The model under review builds one solid part; all positions refer to its coordinate system, in mm. Face numbers are marked on the shaded views. Give positions to 0.01 mm unless a question says otherwise; leave off trailing zeros. Loops run counter-clockwise (first coordinate to the right, second up) from the corner with the lowest first, then second, coordinate; pieces in that order, holes last. Notation, with made-up numbers: M -34.5,61 L -15.5,61 A16 ccw -15.5,91 Z; hole C -6.75,80.5 d9. An arc over 180 degrees is marked long. Return JSON: item names as keys, results as strings.
```python
from build123d import *

# Parameters (mm, degrees)
F1_DEPTH = 203.2
F2_R     = 3.3782
F3_DEPTH = 3.175
F4_R     = 2.5527
F5_DEPTH = 3.175
F6_R     = 1.259666


with BuildPart() as f1:
    # F0 (on Front) → F1 (new body)
    with BuildSketch(Plane.XZ):
        Polygon((30.434872, 0), (0, 0), (21.520704, 21.520704), (19.27564, 23.765768), (-7.665128, -3.175), (30.434872, -3.175), align=None)
    extrude(amount=F1_DEPTH)

    # F2 (on face) → F3 (cut, through all)
    with BuildSketch(Plane(origin=(-2.245064, 0, 2.245064), x_dir=(0, -1, 0), z_dir=(-0.707107, 0, 0.707107))):
        with Locations((50.8, 11.384872)):
            Circle(F2_R)
        with Locations((152.4, 11.384872)):
            Circle(F2_R)
    extrude(amount=-F3_DEPTH, mode=Mode.SUBTRACT)

    # F4 (on face) → F5 (cut, through all)
    with BuildSketch(Plane(origin=(0, 0, -3.175), x_dir=(1, 0, 0), z_dir=(0, 0, -1))):
        with Locations((17.734872, 152.4)):
            Circle(F4_R)
        with Locations((17.734872, 50.8)):
            Circle(F4_R)
    extrude(amount=-F5_DEPTH, mode=Mode.SUBTRACT)

    # F6
    f6_edges = [f1.edges().sort_by_distance(p)[0] for p in [
        (-7.665128, -101.6, -3.175),
    ]]
    fillet(f6_edges, radius=F6_R)


solid = f1.part
```
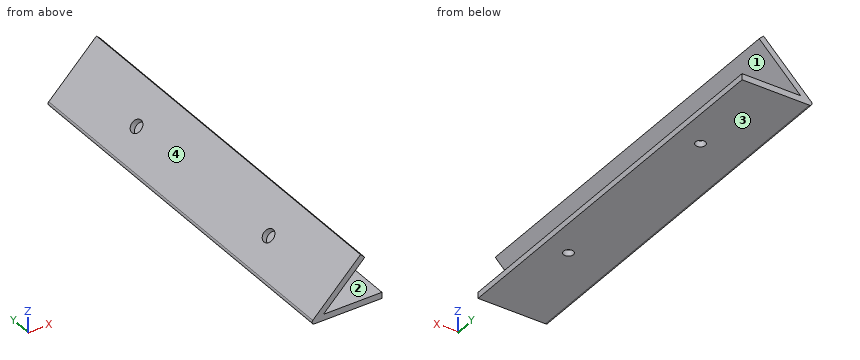
1) Consider section A-A on x = 13.5. Write out the cut boundary in (y, z) (3 decimals).
From the geometry:
{"outline": "M -203.2,-3.175 L 0,-3.175 L 0,0 L -203.2,0 Z; M -203.2,13.5 L 0,13.5 L 0,17.99 L -203.2,17.99 Z"}
2) Consider section C-C on y = -152.4. Write out the cut boundary in (x, z) (1 decimal).
From the geometry:
{"outline": "M -5.5,-1 A1.3 ccw -4.6,-3.2 L 15.2,-3.2 L 15.2,0 L 0,0 L 5.7,5.7 L 3.4,7.9 Z; M 8.2,12.7 L 10.4,10.4 L 21.5,21.5 L 19.3,23.8 Z; M 20.3,-3.2 L 30.4,-3.2 L 30.4,0 L 20.3,0 Z"}
3) Insertion check: pin 1 (1 mm diameter, centred on x = 3, z = 10.5, fed in from +Y); pin 2 (6 mm diameter, centred on y = -137, z = 5.5, fed in from +X); pin 3 (3 mm diameter, centred on y = -58, z = 6.5, fed in from -X); pin 4 (6 mm diameter, centred on y = -42, z = 11, fed in from +X). Each pin has a flat end and moves straight along its axis. Give the tip position at first contact, or say it passes through.
From the geometry:
{"pin 1": "through", "pin 2": "x = 8.5", "pin 3": "x = 0.51", "pin 4": "x = 14"}
4) Wall thickness on L1, parallel to X at y = -50.8, z = -1.65; L2, parallel to X at y = -152.4, z = -1; L3, parallel to X at y = -109, z = -1.75: over which ranges is each line inside the solid? List them lowest first. Write a range as from..to.
From the geometry:
{"L1": "-5.86..15.18, 20.29..30.43", "L2": "-5.49..15.18, 20.29..30.43", "L3": "-5.87..30.43"}
5) The part is to be moulded in two halves that separate along Z. For the marked faces 1, 2, 3 and 4, say which applies: released by +Z, released by -Z, zero draft, split by the parting line, or undercut.
From the geometry:
{"face 1": "undercut", "face 2": "undercut", "face 3": "released by -Z", "face 4": "released by +Z"}
6) Consider section B-B on y = -39.5. Write out the cut boundary in (x, z) (3 decimals), then the cut area to 3 significant figures.
From the geometry:
{"outline": "M -5.515,-1.025 A1.26 ccw -4.624,-3.175 L 30.435,-3.175 L 30.435,0 L 0,0 L 21.521,21.521 L 19.276,23.766 Z", "area": "216 mm²"}
7) Consider section D-D on x = 25.5. Write out the cut boundary in (y, z) (3 decimals).
From the geometry:
{"outline": "M -203.2,-3.175 L 0,-3.175 L 0,0 L -203.2,0 Z"}
